Here's how the part is built. I have some questions about the finished solid (model axes, mm). Face numbers are marked on the shaded views. A direction names the side the tool comes from. Give positions to 0.01 mm unless a question says otherwise; leave off trailing zeros. Order: outer loops, then holes, each group sorted by start corner. A loop starts at its lowest first (then second) coordinate and runs counter-clockwise, first axis right, second up.
from build123d import *

# Parameters (mm, degrees)
BOSS_EXTRUDE1_DEPTH      = 20
BOSS_EXTRUDE1_DEPTH_BACK = 5
BOSS_EXTRUDE2_START      = -5
BOSS_EXTRUDE2_DEPTH      = 5
BOSS_EXTRUDE3_START      = 135
BOSS_EXTRUDE3_DEPTH      = 135


with BuildPart() as part:
    # Sketch1 → Boss-Extrude1 (new, two sides: drawn at the far end of the back side and taken through both)
    with BuildSketch(Plane.XY.offset(-BOSS_EXTRUDE1_DEPTH_BACK)):
        with BuildLine():
            Line((0, 25), (0, 17))
            ThreePointArc((0, 17), (-17, 0), (0, -17))
            Line((0, -17), (0, -25))
            ThreePointArc((0, -25), (-25, 0), (0, 25))
        make_face()
    extrude(amount=BOSS_EXTRUDE1_DEPTH + BOSS_EXTRUDE1_DEPTH_BACK)

    # Sketch2 → Boss-Extrude2 (add)
    with BuildSketch(Plane.XY.offset(BOSS_EXTRUDE2_START)):
        with BuildLine():
            Line((0, 25), (0, 77))
            Line((0, 77), (-65, 77))
            Line((-65, 77), (-65, 32.113081447))
            ThreePointArc((-65, 32.113081447), (-61.581037686, -38.262590053), (0, -72.5))
            Line((0, -72.5), (0, -25))
            ThreePointArc((0, -25), (-25, 0), (0, 25))
        make_face()
    extrude(amount=BOSS_EXTRUDE2_DEPTH)

    # Sketch3 → Boss-Extrude3 (add)
    with BuildSketch(Plane(origin=(0, 0, -5), x_dir=(-1, 0, 0), z_dir=(0, 0, -1)).offset(BOSS_EXTRUDE3_START)):
        with BuildLine():
            Line((60, 30.923292192), (60, 77))
            Line((60, 77), (65, 77))
            Line((65, 77), (65, 32.113081447))
            ThreePointArc((65, 32.113081447), (61.581037686, -38.262590053), (0, -72.5))
            Line((0, -72.5), (0, -67.5))
            ThreePointArc((0, -67.5), (57.634938288, -35.134938288), (60, 30.923292192))
        make_face()
    extrude(amount=-BOSS_EXTRUDE3_DEPTH)

    # Mirror5: part across plane


with BuildPart() as part_1:
    add(part.part)
    add(part.part.mirror(Plane.XY.offset(-140)))


solid = part_1.part
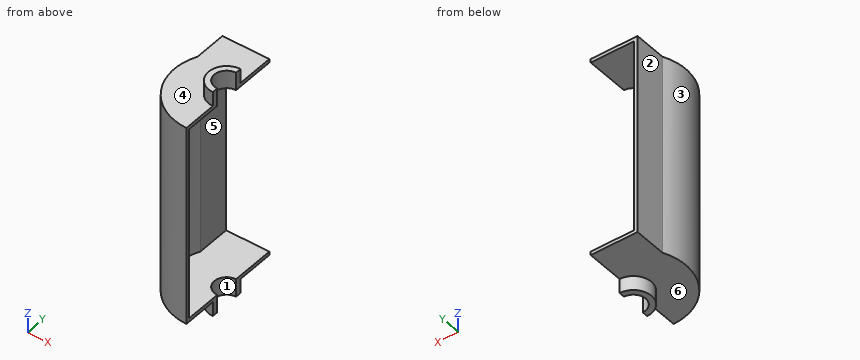
Q1. If we section it at A-A on y = 64.5: List the corners of the cut face in (x, z) for me.
Filled sheet:
outline: (-65, -280) - (0, -280) - (0, -275) - (-60, -275) - (-60, -5) - (0, -5) - (0, 0) - (-65, 0) - close
Q2. If we section it at C-C on z = -180.5: List the corners of the cut face in (x, y) for me.
Filled sheet:
outline: (-65, 32.11) arc R72.5 ccw to (0, -72.5) - (0, -67.5) arc R67.5 cw to (-60, 30.92) - (-60, 77) - (-65, 77) - close
Q3. I need wall thicknesses on L1, parallel to Z at x = -50.5, y = -31; L2, parallel to X at y = 70, z = -146; L3, parallel to Z at x = -62.5, y = 38.5. Which ranges of each line are inside material? Lowest first, please.
Filled sheet:
L1: z = -280 to -275, -5 to 0
L2: x = -65 to -60
L3: z = -280 to 0
Q4. For the marked faces 1 and 2, which set-ups out of +Z, -Z, +X, -X, +Y, -Y let a thin tool reach every point of the face, with its end or its side?
Filled sheet:
face 1: +Z, -Z, +X
face 2: +Z, -Z, -X, +Y
Q5. If we section it at D-D on x = -54: List the corners of the cut face in (y, z) for me, plus the area to 3 significant figures.
Filled sheet:
outline: (-48.38, -280) - (77, -280) - (77, -275) - (-40.5, -275) - (-40.5, -5) - (77, -5) - (77, 0) - (-48.38, 0) - close
area: 3,380 mm2
Q6. If we section it at B-B on x = -7.5: List the corners of the cut face in (y, z) for me.
Filled sheet:
outline: (-72.11, -280) - (-23.85, -280) - (-23.85, -300) - (-15.26, -300) - (-15.26, -275) - (-67.08, -275) - (-67.08, -5) - (-15.26, -5) - (-15.26, 20) - (-23.85, 20) - (-23.85, 0) - (-72.11, 0) - close; (15.26, -300) - (23.85, -300) - (23.85, -280) - (77, -280) - (77, -275) - (15.26, -275) - close; (15.26, -5) - (77, -5) - (77, 0) - (23.85, 0) - (23.85, 20) - (15.26, 20) - close
Q7. Thinking about a two-plate mould opening in Z: for the marked faces 3, 4, 5 and 6, which applies, released by +Z, released by -Z, zero draft, split by the parting line, or undercut?
Filled sheet:
face 3: zero draft
face 4: released by +Z
face 5: undercut
face 6: released by -Z
Q8. I'm going to push flat-ended pins straight in: P1, Ø12, axis at y = 50, z = -58, coming from the -X side; P2, Ø5, axis at y = -43, z = -243, coming from the +X side; P3, Ø1.5, axis at y = -47.5, z = -88.5, coming from the -X side. Where does each tip first touch, or does it pass through?
Filled sheet:
P1: stops at x = -65
P2: stops at x = -49.86
P3: stops at x = -55.41
